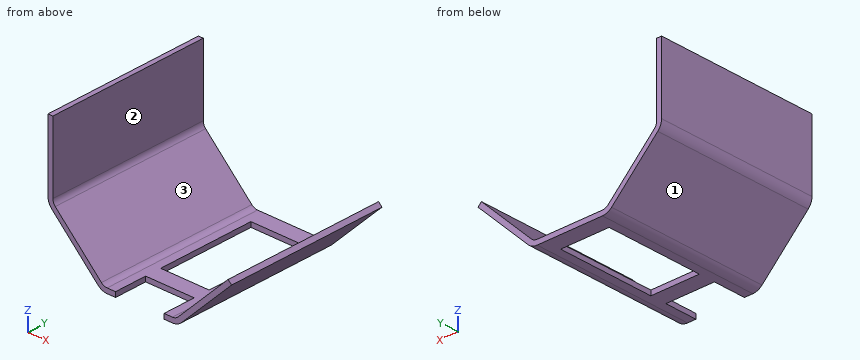
Autodesk Inventor part; units mm, degrees
ref_plane "YZ Plane" through (0, 0, 0) normal (1, 0, 0) x (0, 1, 0)
ref_plane "XZ Plane" through (0, 0, 0) normal (0, 1, 0) x (-1, 0, 0)
ref_plane "XY Plane" through (0, 0, 0) normal (0, 0, 1) x (1, 0, 0)
sketch "Sketch1" plane through (0, 0, 0) normal (0, 0, 1) x (1, 0, 0)
  line L0 (-23.5, -50) -> (23.5, -50)
  line L1 (23.5, -50) -> (23.5, 50)
  line L2 (23.5, 50) -> (-23.5, 50)
  line L3 (-23.5, 50) -> (-23.5, -50)
  line L4 (-23.5, -50) -> (23.5, 50) construction
  line L5 (23.5, -50) -> (-23.5, 50) construction
  point P0 (0, 0)
  dimension "d154" = 47
  dimension "d155" = 100
extrude "Plate3" add sketch "Sketch1" along normal blind 3
sketch "Sketch7" plane through (21.3787, 50, 2.1213) normal (0.7071068, 0, -0.7071068) x (0, 1, 0)
  line L0 (-100, 0) -> (0, 0)
  line L1 (0, 0) -> (0, 47)
  line L2 (0, 47) -> (-100, 47)
  line L3 (-100, 47) -> (-100, 0)
edge flange "Flange3" height 47 angle 45 thickness 3 bend radius 5 thickness toward (0.7071068, 0, -0.7071068) relief round relief width 3 relief depth 1.5 corner gap 5 corner form 0 edges at (23.5, 0, 3) (-23.5, 0, 3) wall of the first edge with corners at (21.3787, -50, 2.1213) (21.3787, 50, 2.1213) (54.6127, 50, 35.3553) (54.6127, -50, 35.3553)
bend "Bend3"
corner "Corner3"
sketch "Sketch8" plane through (0, 0, 3) normal (0, 0, 1) x (1, 0, 0)
  line L0 (15, 40) -> (-15, 40)
  line L1 (-15, 40) -> (-15, -20)
  line L2 (-15, -20) -> (15, -20)
  line L3 (15, -20) -> (15, 40)
  line L4 (15, 40) -> (-15, -20) construction
  line L5 (-15, 40) -> (15, -20) construction
  line L6 (-23.5, 50) -> (20.1863, 50)
  line L7 (-20.1863, -50) -> (20.1863, -50)
  line L8 (15, -50) -> (-15, -50)
  line L9 (-15, -50) -> (-15, -30)
  line L10 (-15, -30) -> (15, -30)
  line L11 (15, -30) -> (15, -50)
  point P0 (0, 0)
  point P1 (0, 10)
  point P2 (-15, -50)
  dimension "d166" = 30
  dimension "d168" = 10
  dimension "d182" = 10
  dimension "d183" = 20
extrude "Cut1" cut sketch "Sketch8" against normal blind 3
sketch "Sketch9" plane through (-53.734, -50, 33.234) normal (-1, 0, 0) x (0, -1, 0)
  line L0 (-100, 0) -> (0, 0)
  line L1 (0, 0) -> (0, 46)
  line L2 (0, 46) -> (-100, 46)
  line L3 (-100, 46) -> (-100, 0)
edge flange "Flange4" height 46 angle 45 thickness 3 bend radius 5 thickness toward (-1, 0, 0) relief round relief width 3 relief depth 1.5 edges at (-54.6127, 0, 35.3553) wall of the first edge with corners at (-53.734, 50, 33.234) (-53.734, -50, 33.234) (-53.734, -50, 79.234) (-53.734, 50, 79.234)
bend "Bend4"
corner "Corner4"
properties part number "DS-B-101 Axis" material "Stainless Steel"
Can you work these out from the model? Positions are in its coordinate system, mm. Face numbers are marked on the shaded views. Give positions to 0.01 mm unless a question says otherwise; leave off trailing zeros. Loops run counter-clockwise (first coordinate to the right, second up) from the corner with the lowest first, then second, coordinate; pieces in that order, holes last. Notation, with made-up numbers: M -18.75,-2.5 L 5.25,-2.5 A14 ccw 5.25,19.5 Z; hole C 50.25,-27 d1. An arc over 180 degrees is marked long. Answer in a Markdown table with one row per item.
1. Suppose I cut it at D-D on x = -17.5. Write out the boundary of the cut face in (y, z).
Taken from the geometry:
| item | result |
|---|---|
| outline | M -50,0 L 50,0 L 50,3 L -50,3 Z |
2. Suppose I cut it at A-A on y = -38. Write out the boundary of the cut face in (x, z), plus the area to 3 significant figures.
Taken from the geometry:
| item | result |
|---|---|
| outline | M -56.73,36.55 A8 ccw -54.39,30.89 L -25.84,2.34 A8 ccw -20.19,0 L -15,0 L -15,3 L -20.19,3 A5 cw -23.72,4.46 L -52.27,33.01 A5 cw -53.73,36.55 L -53.73,79.23 L -56.73,79.23 Z; M 15,0 L 20.19,0 A8 ccw 25.84,2.34 L 56.73,33.23 L 54.61,35.36 L 23.72,4.46 A5 cw 20.19,3 L 15,3 Z |
| area | 457 mm² |
3. Suppose I cut it at B-B on x = -1.5. Write out the boundary of the cut face in (y, z), plus the area to 3 significant figures.
Taken from the geometry:
| item | result |
|---|---|
| outline | M -30,0 L -20,0 L -20,3 L -30,3 Z; M 40,0 L 50,0 L 50,3 L 40,3 Z |
| area | 60.0 mm² |
4. For pin 1 Ø2 at (y, z) = (-19, 51.5) entering from +X; pin 2 Ø3.5 at (x, z) = (3.5, 2) entering from -Y; pin 3 Ø20 at (x, y) = (8.5, 0.5) entering from +Z, each with a flat end and sliding along its axis, tell me the tip position at first contact or that it passes through.
Taken from the geometry:
| item | result |
|---|---|
| pin 1 | stops at x = -53.73 |
| pin 2 | stops at y = -30 |
| pin 3 | stops at z = 3 |
5. Thinking about a two-plate mould opening in X: for the marked faces 1, 2 and 3, which applies, released by +X, released by -X, zero draft, split by the parting line, or undercut?
Taken from the geometry:
| item | result |
|---|---|
| face 1 | released by -X |
| face 2 | released by +X |
| face 3 | undercut |
6. Suppose I cut it at C-C on z = 9. Write out the boundary of the cut face in (x, y).
Taken from the geometry:
| item | result |
|---|---|
| outline | M -32.5,-50 L -28.26,-50 L -28.26,50 L -32.5,50 Z; M 28.26,-50 L 32.5,-50 L 32.5,50 L 28.26,50 Z |
7. If I drill on line 1 along X through (y, z) = (25, 48.5); line 2 along X through (y, z) = (-2, 22); line 3 along X through (y, z) = (34, 13), over which ranges is the centre line in solid material (lowest first)?
Taken from the geometry:
| item | result |
|---|---|
| line 1 | x = -56.73 to -53.73 |
| line 2 | x = -45.5 to -41.26, 41.26 to 45.5 |
| line 3 | x = -36.5 to -32.26, 32.26 to 36.5 |
